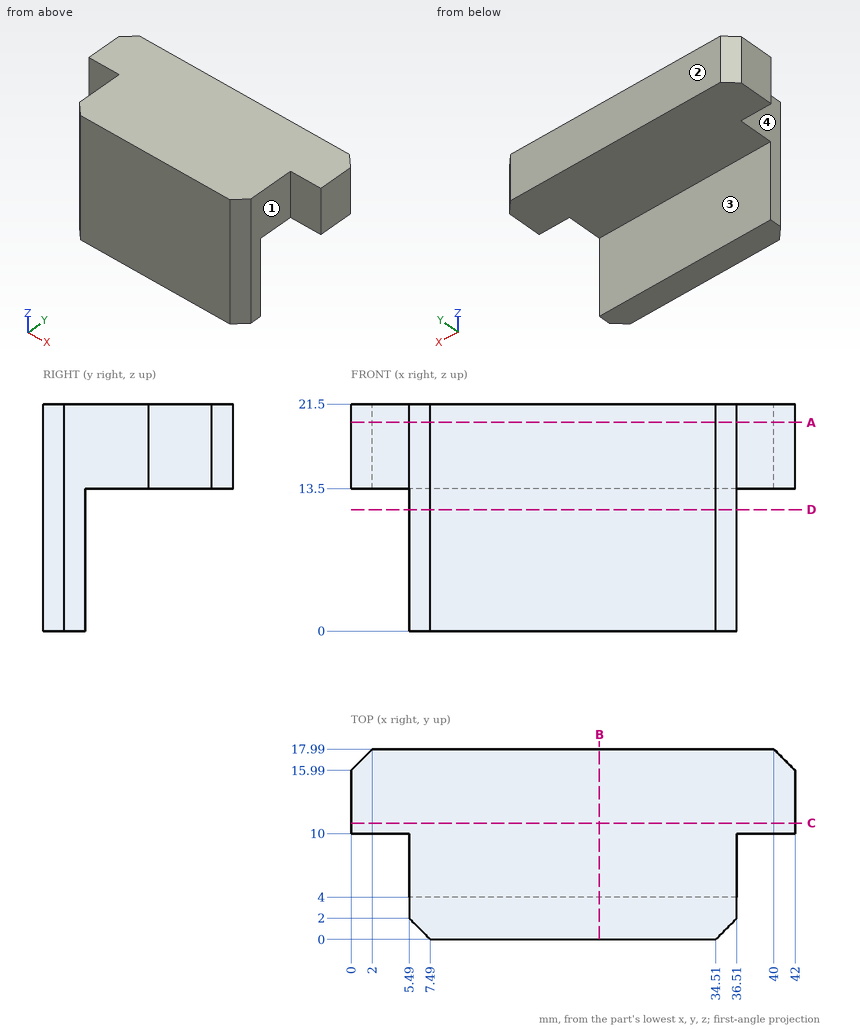
For this review, use the dimensioned drawing (mm, ordinates from the lowest corner) and the shaded views. A direction names the side the tool comes from. Coordinates: 2 decimals unless noted, no trailing zeros. Loops run counter-clockwise (first coordinate to the right, second up) from the corner with the lowest first, then second, coordinate; pieces in that order, holes last. Notation, with made-up numbers: (73, -33) -> (127, -33) arc R36 ccw to (127, 5) -> close; hole circle Ø4 at (-7.75, 63.5). An arc over 180 degrees is marked (long way). Return JSON: item names as keys, results as strings. Group by question number.
(1) To check wall thickness, follow L1, parallel to Y at x = 21, z = 8.5; L2, parallel to X at y = 2.25, z = 17.75; L3, parallel to Z at x = 26.5, y = 6.75. State the ranges of each line that lie inside material, in increasing order.
(2) For pin 1 Ø4.5 at (x, z) = (3, 16) entering from -Y; pin 2 Ø5 at (x, y) = (31.5, 11.5) entering from -Z; pin 3 Ø5 at (x, z) = (6.5, 10.5) entering from +Y, all flat-tipped, find the tip position at first contact; note any pin that passes through.
(3) Consider section B-B, the plane x = 23.5. Give the boundary of the cut face in (y, z).
(4) Consider section D-D, the plane z = 11.5. Give the boundary of the cut face in (x, y), plus the area to 3 significant figures.
(5) Tool access review of the marked faces 1, 2, 3 and 4: name each direction out of +Z, -Z, +X, -X, +Y, -Y from which nothing blocks a thin tool from reaching the whole face with its end or side.
(6) Consider section C-C, the plane y = 11. Give the boundary of the cut face in (x, z), plus the area to 3 significant figures.
(7) Consider section A-A, the plane z = 19.75. Give the boundary of the cut face in (x, y).
Results below:
{
 "1": {"L1": "y = 0 to 4", "L2": "x = 5.49 to 36.51", "L3": "z = 13.5 to 21.5"},
 "2": {"pin 1": "stops at y = 10", "pin 2": "stops at z = 13.5", "pin 3": "stops at y = 4"},
 "3": {"outline": "(0, 0) -> (4, 0) -> (4, 13.5) -> (17.99, 13.5) -> (17.99, 21.5) -> (0, 21.5) -> close"},
 "4": {"outline": "(5.49, 2) -> (7.49, 0) -> (34.51, 0) -> (36.51, 2) -> (36.51, 4) -> (5.49, 4) -> close", "area": "120 mm2"},
 "5": {"face 1": "+Z, -Z, +X, -Y", "face 2": "+Z, -Z, +X, -X, +Y", "face 3": "-Z, +X, -X, +Y", "face 4": "+Z, -Z, -X, -Y"},
 "6": {"outline": "(0, 13.5) -> (42, 13.5) -> (42, 21.5) -> (0, 21.5) -> close", "area": "336 mm2"},
 "7": {"outline": "(0, 10) -> (5.49, 10) -> (5.49, 2) -> (7.49, 0) -> (34.51, 0) -> (36.51, 2) -> (36.51, 10) -> (42, 10) -> (42, 15.99) -> (40, 17.99) -> (2, 17.99) -> (0, 15.99) -> close"}
}
